Check sheet for the modelled part. Datum: model origin and axes. Units: mm. Round coordinates to 2 decimals unless told otherwise and drop trailing zeros. Loops run counter-clockwise (first coordinate to the right, second up) from the corner with the lowest first, then second, coordinate; pieces in that order, holes last. Notation, with made-up numbers: (33, 41.25) - (47, 41.25) arc R9 cw to (47, 54.25) - close; hole circle Ø8 at (38.5, 89). An arc over 180 degrees is marked (long way). Answer in a Markdown table with one row per item. Add a question column.
(1) Cross-section at B-B on y = 126. Enter the section's corners in (x, z), then the cut area to 3 significant figures.
(2) Cross-section at A-A on z = 0.95. Enter the section's corners in (x, y), then the cut area to 3 significant figures.
(3) Gauge pin test, flat ends, axial feed: pin 1 (0.9 mm diameter, centred on x = -19, z = 2, fed in from +Y); pin 2 (1.5 mm diameter, centred on x = 3.5, z = 1, fed in from -Y); pin 3 (0.9 mm diameter, centred on y = 182.5, z = 1.5, fed in from -X). Record the tip position at first contact, or that the pin passes through.
(4) Cross-section at C-C on y = 189.5. Enter the section's corners in (x, z).
(5) Thickness scan on line 1 along Y through (x, z) = (-18.75, 2.75); line 2 along X through (y, z) = (106.5, 1.8); line 3 along X through (y, z) = (127.5, 0.65). Record the ranges inside material, lowest first.
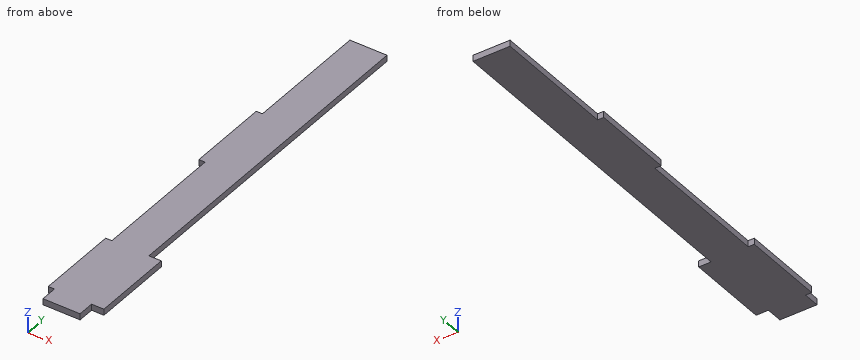
from build123d import *

# Parameters (mm, degrees)
SKETCH1_W           = 18
SKETCH1_H           = 61
BASE_SHAPE_DEPTH    = 3
SKETCH2_W           = 6
SKETCH2_H           = 40
SKETCH2_W_2         = 3
FINGERS_DEPTH       = 3
SKETCH3_W           = 18
SKETCH3_H           = 3
BOSS_EXTRUDE1_DEPTH = 153
SKETCH4_W           = 3
SKETCH4_H           = 40
BOSS_EXTRUDE3_DEPTH = 3


with BuildPart() as part:
    # Sketch1 → Base Shape (new body)
    with BuildSketch(Plane.XY):
        with Locations((-9, 30.5)):
            Rectangle(SKETCH1_W, SKETCH1_H)
    extrude(amount=BASE_SHAPE_DEPTH)

    # Sketch2 → Fingers (add)
    with BuildSketch(Plane.XY.offset(3)):
        with Locations((3, 28)):
            Rectangle(SKETCH2_W, SKETCH2_H)
        with Locations((-19.5, 28)):
            Rectangle(SKETCH2_W_2, SKETCH2_H)
    extrude(amount=-FINGERS_DEPTH)

    # Sketch3 → Boss-Extrude1 (add)
    with BuildSketch(Plane(origin=(0, 61, 0), x_dir=(1, 0, 0), z_dir=(0, 1, 0))):
        with Locations((-9, -1.5)):
            Rectangle(SKETCH3_W, SKETCH3_H)
    extrude(amount=BOSS_EXTRUDE1_DEPTH)

    # Sketch4 → Boss-Extrude3 (add, through all)
    with BuildSketch(Plane.XY.offset(3)):
        with Locations((-19.5, 133)):
            Rectangle(SKETCH4_W, SKETCH4_H)
    extrude(amount=-BOSS_EXTRUDE3_DEPTH)


solid = part.part
Answers:
| question | item | result |
|---|---|---|
| 1 | outline | (-21, 0) - (0, 0) - (0, 3) - (-21, 3) - close |
| 1 | area | 63.0 mm^2 |
| 2 | outline | (-21, 8) - (-18, 8) - (-18, 0) - (0, 0) - (0, 8) - (6, 8) - (6, 48) - (0, 48) - (0, 214) - (-18, 214) - (-18, 153) - (-21, 153) - (-21, 113) - (-18, 113) - (-18, 48) - (-21, 48) - close |
| 2 | area | 4,330 mm^2 |
| 3 | pin 1 | stops at y = 153 |
| 3 | pin 2 | stops at y = 8 |
| 3 | pin 3 | stops at x = -18 |
| 4 | outline | (-18, 0) - (0, 0) - (0, 3) - (-18, 3) - close |
| 5 | line 1 | y = 8 to 48, 113 to 153 |
| 5 | line 2 | x = -18 to 0 |
| 5 | line 3 | x = -21 to 0 |
